Build history of the part. All positions in model axes, mm. A direction names the side the tool comes from. Give positions to 0.01 mm unless a question says otherwise; leave off trailing zeros. Write each loop counter-clockwise with the first axis right and the second up, starting at its lowest first coordinate (ties: lowest second). Pieces come first, ordered by that corner, then holes. Notation, with made-up numbers: (36, 3.25) -> (43, 3.25) arc R35 ccw to (43, 40.25) -> close; hole circle Ø11 at (41, 54). An arc over 180 degrees is marked (long way). Put each result on its own line as item: value. Start each with the question number.
Item 1: Flat gauge pin, fed straight in: pin 1 Ø4 at (x, z) = (25.4, 50.8) entering from +Y. Where does the tip first touch, or does it go through?
Item 2: Tool access for faces 1 (the cylindrical face through (12.75, 24.62, 61.01)), 2 (the flat face through (25, 23.812, 31)): list every direction of +Z, -Z, +X, -X, +Y, -Y with a clear straight run to the whole face (end or side of a thin tool).
Item 3: Slice it at A-A, the plane z = 30. List the corners of the cut face in (x, y), plus the area to 3 significant figures.
Item 4: Slice it at B-B, the plane x = 18. List the corners of the cut face in (y, z).
Item 5: Slice it at C-C, the plane y = 21.75. List the corners of the cut face in (x, z).
Item 6: Two-plate mould, pull along Y, no slides. Class faces 3 (the cylindrical face through (50, 14.8, 26.74)), 4 (the cylindrical face through (35.613, 0.805, 12.591)), 5 (the flat face through (25, 1.587, 31)): pulls with the +Y half, pulls with the -Y half, needs draft (parallel to the pull), parting line crosses it, or undercut.
Item 7: Slice it at D-D, the plane x = 38.1. Give the number of separate pieces and of enclosed holes in the cut face, plus the area to 3 significant figures.
Item 8: Drill centre lines: line 1 along X through (y, z) = (25.1, 38.1); line 2 along Z through (x, y) = (38.1, 0.7); line 3 along X through (y, z) = (9, 47). Where is each one in solid material? Low to high.
```python
from build123d import *

# Parameters (mm, degrees)
SKETCH1_W           = 50.8
SKETCH1_H           = 25.4
SKETCH1_W_2         = 47.625
SKETCH1_H_2         = 22.225
BOSS_EXTRUDE1_DEPTH = 63.5
SKETCH2_R           = 2.4892
CUT_EXTRUDE1_DEPTH  = 26.4
SKETCH3_R           = 2.4892
CUT_EXTRUDE2_DEPTH  = 51.8


with BuildPart() as part:
    # Sketch1 → Boss-Extrude1 (new body)
    with BuildSketch(Plane.XY):
        with Locations((25.4, 12.7)):
            Rectangle(SKETCH1_W, SKETCH1_H)
        with Locations((25.4, 12.7)):
            Rectangle(SKETCH1_W_2, SKETCH1_H_2, mode=Mode.SUBTRACT)
    extrude(amount=BOSS_EXTRUDE1_DEPTH)

    # Sketch2 → Cut-Extrude1 (cut, through all)
    with BuildSketch(Plane(origin=(0, 25.4, 0), x_dir=(1, 0, 0), z_dir=(0, 1, 0))):
        with Locations((12.7, -12.7)):
            Circle(SKETCH2_R)
        with Locations((25.4, -12.7)):
            Circle(SKETCH2_R)
        with Locations((38.1, -12.7)):
            Circle(SKETCH2_R)
        with Locations((25.4, -25.4)):
            Circle(SKETCH2_R)
        with Locations((38.1, -25.4)):
            Circle(SKETCH2_R)
        with Locations((25.4, -38.1)):
            Circle(SKETCH2_R)
        with Locations((38.1, -38.1)):
            Circle(SKETCH2_R)
        with Locations((25.4, -50.8)):
            Circle(SKETCH2_R)
        with Locations((38.1, -50.8)):
            Circle(SKETCH2_R)
        with Locations((25.4, -63.5)):
            Circle(SKETCH2_R)
        with Locations((38.1, -63.5)):
            Circle(SKETCH2_R)
        with Locations((12.7, -25.4)):
            Circle(SKETCH2_R)
        with Locations((12.7, -38.1)):
            Circle(SKETCH2_R)
        with Locations((12.7, -50.8)):
            Circle(SKETCH2_R)
        with Locations((12.7, -63.5)):
            Circle(SKETCH2_R)
    extrude(amount=-CUT_EXTRUDE1_DEPTH, mode=Mode.SUBTRACT)

    # Sketch3 → Cut-Extrude2 (cut, through all)
    with BuildSketch(Plane.ZY):
        with Locations((12.7, 12.7)):
            Circle(SKETCH3_R)
        with Locations((25.4, 12.7)):
            Circle(SKETCH3_R)
        with Locations((38.1, 12.7)):
            Circle(SKETCH3_R)
        with Locations((50.8, 12.7)):
            Circle(SKETCH3_R)
        with Locations((63.5, 12.7)):
            Circle(SKETCH3_R)
    extrude(amount=-CUT_EXTRUDE2_DEPTH, mode=Mode.SUBTRACT)


solid = part.part
```
Values follow:
1. pin 1: through
2. face 1: +Z, +Y, -Y
2. face 2: +Z, -Z
3. outline: (0, 0) -> (50.8, 0) -> (50.8, 25.4) -> (0, 25.4) -> close; hole (1.59, 1.59) -> (49.21, 1.59) -> (49.21, 23.81) -> (1.59, 23.81) -> close
3. area: 232 mm2
4. outline: (0, 0) -> (1.59, 0) -> (1.59, 63.5) -> (0, 63.5) -> close; (23.81, 0) -> (25.4, 0) -> (25.4, 63.5) -> (23.81, 63.5) -> close
5. outline: (0, 0) -> (1.59, 0) -> (1.59, 63.5) -> (0, 63.5) -> close; (49.21, 0) -> (50.8, 0) -> (50.8, 63.5) -> (49.21, 63.5) -> close
6. face 3: undercut
6. face 4: needs draft
6. face 5: undercut
7. separate pieces: 10
7. enclosed holes: 0
7. area: 130 mm2
8. line 1: 0 to 10.21, 15.19 to 22.91, 27.89 to 35.61, 40.59 to 50.8
8. line 2: 0 to 10.21, 15.19 to 22.91, 27.89 to 35.61, 40.59 to 48.31, 53.29 to 61.01
8. line 3: 0 to 1.59, 49.21 to 50.8
